Design review of the part built by this model. Coordinates are the model's own, in mm. A direction names the side the tool comes from. Round coordinates to 2 decimals unless told otherwise and drop trailing zeros. Write each loop counter-clockwise with the first axis right and the second up, starting at its lowest first coordinate (ties: lowest second). Pieces come first, ordered by that corner, then holes. Notation, with made-up numbers: M 42,71.5 L 89,71.5 A36 ccw 89,108.5 Z; hole C 39.25,28 d9. An arc over 180 degrees is marked long. Use CSV: the item, a comma, the result in double quotes.
from build123d import *

# Parameters (mm, degrees)
F0_W     = 1219.2
F0_H     = 762
F1_DEPTH = 6.35
F2_W     = 50.8
F2_H     = 50.8
F3_DEPTH = 768.35
F4_W     = 546.1
F4_H     = 50.8
F5_DEPTH = 50.8
F7_W     = 1041.4
F7_H     = 50.8
F8_DEPTH = 50.8


with BuildPart() as f1:
    # F0 (on Top) → F1 (new body)
    with BuildSketch(Plane.XY):
        Rectangle(F0_W, F0_H)
    extrude(amount=F1_DEPTH)

    # F2 (on face) → F3 (join)
    with BuildSketch(Plane(origin=(0, 0, 0), x_dir=(1, 0, 0), z_dir=(0, 0, -1))):
        with Locations((546.1, -298.45)):
            Rectangle(F2_W, F2_H)
        with Locations((-546.1, -298.45)):
            Rectangle(F2_W, F2_H)
        with Locations((546.1, 298.45)):
            Rectangle(F2_W, F2_H)
        with Locations((-546.1, 298.45)):
            Rectangle(F2_W, F2_H)
    extrude(amount=F3_DEPTH)

    # F4 (on face) → F5 (join)
    with BuildSketch(Plane(origin=(-571.5, 0, 0), x_dir=(0, -1, 0), z_dir=(-1, 0, 0))):
        with Locations((0, -425.45)):
            Rectangle(F4_W, F4_H)
    extrude(amount=-F5_DEPTH)

    # F6: F1 across plane


with BuildPart() as f1_1:
    add(f1.part)
    add(f1.part.mirror(Plane.YZ))

    # F7 (on face) → F8 (join, through all)
    with BuildSketch(Plane(origin=(0, 0, -450.85), x_dir=(1, 0, 0), z_dir=(0, 0, -1))):
        Rectangle(F7_W, F7_H)
    extrude(amount=-F8_DEPTH)


solid = f1_1.part
1) Add section C-C on y = 73. Write out the cut boundary in (x, z), then the cut area to 3 significant figures.
Answers:
outline,"M -609.6,0 L 609.6,0 L 609.6,6.35 L -609.6,6.35 Z; M -571.5,-450.85 L -520.7,-450.85 L -520.7,-400.05 L -571.5,-400.05 Z; M 520.7,-450.85 L 571.5,-450.85 L 571.5,-400.05 L 520.7,-400.05 Z"
area,"12,900 mm²"
2) Machinability: for faces 1 (the face through (-520.7, -273, -411)), 2 (the face through (546, -323.85, -379)), 3 (the face through (546, 273.05, -197)), 4 (the face through (-520.7, 264, -411)), 5 (the face through (-3, 1, -450.85)), which of the approach directions +Z, -Z, +X, -X, +Y, -Y give a long, thin tool a straight path to every point of the face, cutting with its end or side? Answer none if there is none.
Answers:
face 1,"-Z, -Y"
face 2,"-Z, +X, -X, -Y"
face 3,"+X, -X"
face 4,"-Z, +Y"
face 5,"-Z, +X, -X"
3) Wall thickness on line 1 along X through (y, z) = (-289.5, -336.5); line 2 along Z through (x, y) = (-369, 21.5); line 3 along Y through (x, z) = (-353, -419): over which ranges is each line inside the solid? List them lowest first. Write a range as [from, to].
Answers:
line 1,"[-571.5, -520.7], [520.7, 571.5]"
line 2,"[-450.85, -400.05], [0, 6.35]"
line 3,"[-25.4, 25.4]"
4) Add section B-B on x = -159. Write out the cut boundary in (y, z).
Answers:
outline,"M -381,0 L 381,0 L 381,6.35 L -381,6.35 Z; M -25.4,-450.85 L 25.4,-450.85 L 25.4,-400.05 L -25.4,-400.05 Z"
5) Add section D-D on y = 287.5. Write out the cut boundary in (x, z), then the cut area to 3 significant figures.
Answers:
outline,"M -609.6,0 L -571.5,0 L -571.5,-768.35 L -520.7,-768.35 L -520.7,0 L 520.7,0 L 520.7,-768.35 L 571.5,-768.35 L 571.5,0 L 609.6,0 L 609.6,6.35 L -609.6,6.35 Z"
area,"85,800 mm²"
6) The part is to be moulded in two halves that separate along Y. For faces 6 (the face through (-546, -273.05, -197)), 7 (the face through (-546, 323.85, -379)), 8 (the face through (520.7, -273, -411)), say which applies: released by +Y, released by -Y, zero draft, split by the parting line, or undercut.
Answers:
face 6,"undercut"
face 7,"released by +Y"
face 8,"zero draft"
7) Add section A-A on z = -186. Write out the cut boundary in (x, y).
Answers:
outline,"M -571.5,-323.85 L -520.7,-323.85 L -520.7,-273.05 L -571.5,-273.05 Z; M -571.5,273.05 L -520.7,273.05 L -520.7,323.85 L -571.5,323.85 Z; M 520.7,-323.85 L 571.5,-323.85 L 571.5,-273.05 L 520.7,-273.05 Z; M 520.7,273.05 L 571.5,273.05 L 571.5,323.85 L 520.7,323.85 Z"
8) For pin 1 Ø5 at (x, y) = (25, 124) entering from -Z; pin 2 Ø10 at (y, z) = (299.5, -189) entering from +X, all flat-tipped, find the tip position at first contact; note any pin that passes through.
Answers:
pin 1,"z = 0"
pin 2,"x = 571.5"
